from build123d import *

# Parameters (mm, degrees)
SKETCH8_W                   = 63
SKETCH8_H                   = 40
BOSS_EXTRUDE3_DEPTH         = 20
TAP_DRILL_FOR_M5X0_8_TAP2_D = 4.2
FILLET4_R                   = 2
TAP_DRILL_FOR_M5X0_8_TAP3_D = 4.2
FILLET6_R                   = 12


with BuildPart() as part:
    # Sketch8 → Boss-Extrude3 (new body)
    with BuildSketch(Plane.XY):
        with BuildLine():
            Line((63, -43.532093881), (0, -43.532093881))
            Line((0, -43.532093881), (-25.666666667, -63.532093881))
            Line((-25.666666667, -63.532093881), (-13.5, -63.532093881))
            Line((-13.5, -63.532093881), (11.242912026, -52.54839108))
            ThreePointArc((11.242912026, -52.54839108), (31.551767994, -48.24798089), (51.856795198, -52.56643302))
            Line((51.856795198, -52.56643302), (76.5, -63.532093881))
            Line((76.5, -63.532093881), (88.666666667, -63.532093881))
            Line((88.666666667, -63.532093881), (63, -43.532093881))
        make_face()
        with Locations((31.5, -23.532093881)):
            Rectangle(SKETCH8_W, SKETCH8_H)
        Polygon((-13.5, -63.532093881), (-25.666666667, -63.532093881), (-38.5, -73.532093881), (-13.5, -73.532093881), align=None)
        Polygon((101.5, -73.532093881), (88.666666667, -63.532093881), (76.5, -63.532093881), (76.5, -73.532093881), align=None)
    extrude(amount=-BOSS_EXTRUDE3_DEPTH)

    # Tap Drill for M5x0.8 Tap2 (through all)
    with Locations(Plane(origin=(0, -73.532093881, 0), x_dir=(-1, 0, 0), z_dir=(0, -1, 0))):
        with Locations((26, 10), (-89, 10)):
            Hole(TAP_DRILL_FOR_M5X0_8_TAP2_D / 2)

    # Fillet4
    fillet4_edges = [part.edges().sort_by_distance(p)[0] for p in [
        (63, -23.532093881, 0),
        (82.25, -58.532093881, 0),
        (-19.25, -58.532093881, 0),
        (0, -23.532093881, 0),
        (0, -23.532093881, -20),
        (82.25, -58.532093881, -20),
        (63, -23.532093881, -20),
        (-19.25, -58.532093881, -20),
    ]]
    fillet(fillet4_edges, radius=FILLET4_R)

    # Tap Drill for M5x0.8 Tap3 (through all)
    with Locations(Plane(origin=(0, -3.532093881, 0), x_dir=(1, 0, 0), z_dir=(0, 1, 0))):
        with Locations((8, 10), (55, 10)):
            Hole(TAP_DRILL_FOR_M5X0_8_TAP3_D / 2)

    # Fillet6
    fillet6_edges = [part.edges().sort_by_distance(p)[0] for p in [
        (76.5, -63.532093881, -10),
        (-13.5, -63.532093881, -10),
    ]]
    fillet(fillet6_edges, radius=FILLET6_R)


solid = part.part
Could you check a few things on this model? Use its own coordinates, in mm. A direction names the side the tool comes from. Round coordinates to 2 decimals unless told otherwise and drop trailing zeros. Loops run counter-clockwise (first coordinate to the right, second up) from the corner with the lowest first, then second, coordinate; pieces in that order, holes last. Notation, with made-up numbers: (64, -19.5) - (106, -19.5) arc R34 ccw to (106, 12.5) - close; hole circle Ø3 at (87, 37.25). An arc over 180 degrees is marked (long way). Write item = value, one per line.
1) On a 3-axis mill with a long thin cutter (end or side, diameter ignored), from which of +Z, -Z, +X, -X, +Y, -Y can I reach the whole of each face in a straight line? I mean faces 1 (the flat face through (0, -24, -10)), 2 (the flat face through (-26.2, -73.532, -7.6)), 3 (the flat face through (60.495, -56.41, -9.86)), 4 (the flat face through (63, -24, -10)), 5 (the flat face through (31, -3.532, -10)). Say none if no direction works.
Computed:
face_1 = +Z, -Z, -X, +Y
face_2 = +Z, -Z, +X, -X, -Y
face_3 = +Z, -Z, -Y
face_4 = +Z, -Z, +X, +Y
face_5 = +Z, -Z, +X, -X, +Y
2) If we mould it in two halves opening along Z, with no side actions, what happens to faces 6 (the flat face through (88.8, -73.532, -7.6)), 7 (the flat face through (31, -38, -20)), 8 (the cylindrical face through (9.548, -29.586, -11.419)), 9 (the flat face through (31, -38, 0))? For each: pulls with the +Z half, pulls with the -Z half, needs draft (parallel to the pull), parting line crosses it, or undercut.
Computed:
face_6 = needs draft
face_7 = pulls with the -Z half
face_8 = undercut
face_9 = pulls with the +Z half
3) Imagine slicing it at C-C (z = -4.75). Please give me the cut outline in (x, y).
Computed:
outline = (-38.5, -73.53) - (-13.5, -73.53) - (-13.5, -71.33) arc R12 cw to (-6.37, -60.37) - (11.24, -52.55) arc R50 cw to (51.86, -52.57) - (69.38, -60.36) arc R12 cw to (76.5, -71.33) - (76.5, -73.53) - (101.5, -73.53) - (63, -43.53) - (63, -3.53) - (0, -3.53) - (0, -43.53) - close
4) Imagine slicing it at B-B (x = 55). Please give me the cut outline in (y, z), and give its area (3 significant figures).
Computed:
outline = (-53.97, -20) - (-3.53, -20) - (-3.53, -12.1) - (-53.97, -12.1) - close; (-53.97, -7.9) - (-3.53, -7.9) - (-3.53, 0) - (-53.97, 0) - close
area = 797 mm2
5) Imagine slicing it at D-D (y = -51). Give the number of separate pieces and of enclosed holes in the cut face, and give its area (3 significant figures).
Computed:
separate_pieces = 2
enclosed_holes = 2
area = 956 mm2
6) I need wall thicknesses on line 1 along X through (y, z) = (-21, -9.75); line 2 along Z through (x, y) = (55, -34); line 3 along X through (y, z) = (-47.5, -9.75). Which ranges of each line are inside material? Lowest first, please. Write a range as from..to.
Computed:
line_1 = 0..5.91, 10.09..52.91, 57.09..63
line_2 = -20..-12.1, -7.9..0
line_3 = -5.09..5.91, 10.09..52.91, 57.09..68.09
7) Imagine slicing it at A-A (y = -26). Please give me the cut outline in (x, z).
Computed:
outline = (0, -18) arc R2 ccw to (2, -20) - (61, -20) arc R2 ccw to (63, -18) - (63, -2) arc R2 ccw to (61, 0) - (2, 0) arc R2 ccw to (0, -2) - close; hole circle Ø4.2 at (8, -10); hole circle Ø4.2 at (55, -10)
8) I'm going to push flat-ended pins straight in: P1, Ø5, axis at y = -26, z = -15, coming from the -X side; P2, Ø1.1, axis at y = -72, z = -10.5, coming from the -X side; P3, Ø1.8, axis at y = -72, z = -6, coming from the +X side; P4, Ø8, axis at x = 69, y = -48, coming from the -Z side. Where does each tip first touch, or does it pass through?
Computed:
P1 = 0
P2 = -37.24
P3 = 100.69
P4 = -20
